from build123d import *

# Parameters (mm, degrees)
SKETCH_1_W          = 15
SKETCH_1_H          = 20
SKETCH_1_W_2        = 13
SKETCH_1_H_2        = 18
EXTRUDE_1_DEPTH     = 240
SKETCH_3_R          = 1.6
CUT_EXTRUDE_2_DEPTH = 242.29857024


with BuildPart() as part:
    # 草图1 → 拉伸-薄壁1 (new body)
    with BuildSketch(Plane.XY):
        with Locations((7.5, -10)):
            Rectangle(SKETCH_1_W, SKETCH_1_H)
        with Locations((7.5, -10)):
            Rectangle(SKETCH_1_W_2, SKETCH_1_H_2, mode=Mode.SUBTRACT)
    extrude(amount=EXTRUDE_1_DEPTH)

    # 草图3 → 切除-拉伸2 (cut, through all)
    with BuildSketch(Plane(origin=(0, 0, 0), x_dir=(1, 0, 0), z_dir=(0, 1, 0))):
        with Locations(Location((7.5, -10, 0), (0, 0, 270))):
            Circle(SKETCH_3_R)
        with Locations(Location((7.5, -230, 0), (0, 0, 270))):
            Circle(SKETCH_3_R)
    extrude(amount=-CUT_EXTRUDE_2_DEPTH, mode=Mode.SUBTRACT)


solid = part.part
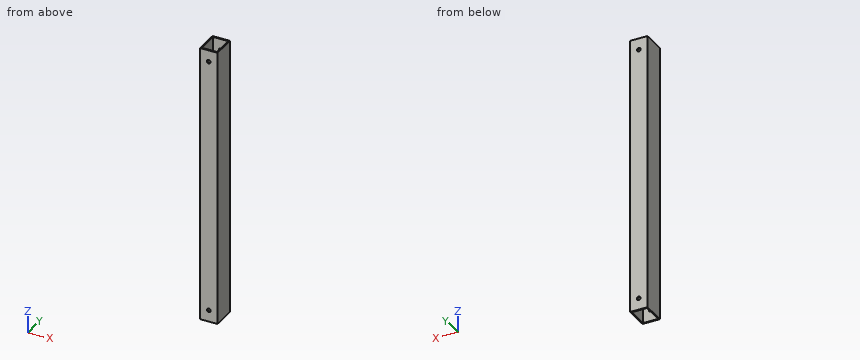
The listing builds one solid part. Answer for the finished solid, in the listing's coordinates (mm). Give positions to 0.01 mm unless a question says otherwise; leave off trailing zeros. Order: outer loops, then holes, each group sorted by start corner. A loop starts at its lowest first (then second) coordinate and runs counter-clockwise, first axis right, second up. Notation, with made-up numbers: (85.5, -4.75) - (131.5, -4.75) arc R11 cw to (131.5, 5.25) - close; hole circle Ø9 at (4, -37.5). An arc over 180 degrees is marked (long way). One line per item, written item: value. Start each with the question number.
1) Given pin 1 Ø1.5 at (x, y) = (5, -3.5) entering from +Z; pin 2 Ø8 at (y, z) = (-7, 202) entering from -X, each flat-ended and moving along its own axis, determine where each tip first touches the part or whether it passes through.
2) A cutting plane is placed at A-A on x = 12. Give the vertices of the cut face in (y, z), then the cut area to 3 significant figures.
3) A cutting plane is placed at C-C on z = 85. Give the vertices of the cut face in (x, y).
4) Find the intervals of material crossed by L1, parallel to Y at x = 9.75, z = 156.5; L2, parallel to X at y = -4.75, z = 206; L3, parallel to X at y = -19.3, z = 230, in increasing order.
5) A cutting plane is placed at B-B on y = -7. Give the vertices of the cut face in (x, z).
Answer sheet:
1. pin 1: passes through
1. pin 2: stops at x = 0
2. outline: (-20, 0) - (-19, 0) - (-19, 240) - (-20, 240) - close; (-1, 0) - (0, 0) - (0, 240) - (-1, 240) - close
2. area: 480 mm2
3. outline: (0, -20) - (15, -20) - (15, 0) - (0, 0) - close; hole (1, -19) - (14, -19) - (14, -1) - (1, -1) - close
4. L1: y = -20 to -19, -1 to 0
4. L2: x = 0 to 1, 14 to 15
4. L3: x = 0 to 5.9, 9.1 to 15
5. outline: (0, 0) - (1, 0) - (1, 240) - (0, 240) - close; (14, 0) - (15, 0) - (15, 240) - (14, 240) - close
